Verification items for the finished model (mm, model axes). Coordinates: 2 decimals unless noted, no trailing zeros. Write each loop counter-clockwise with the first axis right and the second up, starting at its lowest first coordinate (ties: lowest second). Pieces come first, ordered by that corner, then holes. Notation, with made-up numbers: (60, 56) -> (115, 56) arc R12 ccw to (115, 60) -> close; hole circle Ø6 at (53, -11.75). An arc over 180 degrees is marked (long way). Answer in a Markdown table with one row per item.
Autodesk Inventor part; units mm, degrees
ref_plane "YZ Plane" through (0, 0, 0) normal (1, 0, 0) x (0, 1, 0)
ref_plane "XZ Plane" through (0, 0, 0) normal (0, 1, 0) x (-1, 0, 0)
ref_plane "XY Plane" through (0, 0, 0) normal (0, 0, 1) x (1, 0, 0)
sketch "Sketch2" plane through (0, 0, 0) normal (0, 0, 1) x (1, 0, 0)
  circle A0 centre (7.019, 0.1365) radius 2.125
  circle A1 centre (7.019, 0.1365) radius 2.375
  line L0 (7.019, 0.1365) -> (7.019, 4.1365)
  line L1 (7.019, 4.1365) -> (3.019, 4.1365)
  line L2 (3.019, 4.1365) -> (31.019, 4.1365)
  line L3 (31.019, 4.1365) -> (31.019, -3.8635)
  line L4 (31.019, -3.8635) -> (3.019, -3.8635)
  line L5 (3.019, -3.8635) -> (3.019, 4.1365)
  line L6 (17.019, 4.1365) -> (17.019, 2)
  circle A2 centre (27.019, 0.1365) radius 2.375
  point P0 (0, 0)
  dimension "d0" = 4.75
  dimension "d1" = 4
  dimension "d2" = 4
  dimension "d3" = 28
  dimension "d4" = 8
extrude "Extrusion1" add sketch "Sketch2" along normal blind 1.5 contours L2 L3 L4 L5 L1
properties part number "Connector"
1. Sectioned sample at C-C, the plane z = 0.9. Count the separate pieces of the cut face and the enclosed holes in it, and give its area (3 significant figures).
Findings below:
| item | result |
|---|---|
| separate pieces | 1 |
| enclosed holes | 2 |
| area | 189 mm² |
2. Material ranges on probe 1 along X at (y, z) = (0, 0.9); probe 2 along X at (y, z) = (2, 1.2); probe 3 along Y at (x, z) = (29, 0.45), recorded low to high. Write a range as from..to.
Findings below:
| item | result |
|---|---|
| probe 1 | x = 3.02..4.65, 9.39..24.65, 29.39..31.02 |
| probe 2 | x = 3.02..5.55, 8.49..25.55, 28.49..31.02 |
| probe 3 | y = -3.86..-1.17, 1.45..4.14 |
3. Go/stop test with a flat-tipped pin: pin 1 (3 mm diameter, centred on x = 27.02, y = 0.14, fed in from -Z). Record where the tip stops, or that it passes through.
Findings below:
| item | result |
|---|---|
| pin 1 | passes through |
4. Sectioned sample at D-D, the plane x = 25.25. Record the cut outline in (y, z).
Findings below:
| item | result |
|---|---|
| outline | (-3.86, 0) -> (-1.45, 0) -> (-1.45, 1.5) -> (-3.86, 1.5) -> close; (1.72, 0) -> (4.14, 0) -> (4.14, 1.5) -> (1.72, 1.5) -> close |
5. Release check for a two-part mould opening along Y. For faces 1 (the face through (17, 4.136, 1)), 2 (the face through (31.019, 0, 1)), 3 (the face through (25.134, 1.582, 0.74)), 4 (the face through (17, -3.864, 1)) record: released by +Y, released by -Y, zero draft, split by the parting line, or undercut.
Findings below:
| item | result |
|---|---|
| face 1 | released by +Y |
| face 2 | zero draft |
| face 3 | undercut |
| face 4 | released by -Y |
6. Sectioned sample at A-A, the plane x = 5. Record the cut outline in (y, z).
Findings below:
| item | result |
|---|---|
| outline | (-3.86, 0) -> (-1.11, 0) -> (-1.11, 1.5) -> (-3.86, 1.5) -> close; (1.39, 0) -> (4.14, 0) -> (4.14, 1.5) -> (1.39, 1.5) -> close |
7. Sectioned sample at B-B, the plane y = 1.25. Record the cut outline in (x, z), and give its area (3 significant figures).
Findings below:
| item | result |
|---|---|
| outline | (3.02, 0) -> (4.92, 0) -> (4.92, 1.5) -> (3.02, 1.5) -> close; (9.12, 0) -> (24.92, 0) -> (24.92, 1.5) -> (9.12, 1.5) -> close; (29.12, 0) -> (31.02, 0) -> (31.02, 1.5) -> (29.12, 1.5) -> close |
| area | 29.4 mm² |
